```python
from build123d import *

# Parameters (mm, degrees)
SKETCH1_R           = 15
BOSS_EXTRUDE1_DEPTH = 15
SKETCH2_W           = 2.7
SKETCH2_H           = 7.4
SKETCH2_W_2         = 1.7
SKETCH2_H_2         = 6.4
CUT_EXTRUDE1_DEPTH  = 5


with BuildPart() as part:
    # Sketch1 → Boss-Extrude1 (new body)
    with BuildSketch(Plane(origin=(0, 0, 0), x_dir=(1, 0, 0), z_dir=(0, 1, 0))):
        with Locations(Location((0, 0, 0), (0, 0, 270))):
            Circle(SKETCH1_R)
    extrude(amount=BOSS_EXTRUDE1_DEPTH)

    # Sketch2 → Cut-Extrude1 (cut)
    # profile 1 of 3: a face of its own
    with BuildSketch(Plane.XZ):
        with Locations((-11.35, 0)):
            Rectangle(SKETCH2_W, SKETCH2_H)
        with Locations((-11.35, 0)):
            Rectangle(SKETCH2_W_2, SKETCH2_H_2, mode=Mode.SUBTRACT)
    # profile 2 of 3: a face of its own
    with BuildSketch(Plane.XZ):
        with Locations((-11.35, 0)):
            Rectangle(SKETCH2_W_2, SKETCH2_H_2)
    # profile 3 of 3: a face of its own
    with BuildSketch(Plane.XZ):
        with Locations((11.35, 0)):
            Rectangle(SKETCH2_W, SKETCH2_H)
    extrude(amount=-CUT_EXTRUDE1_DEPTH, mode=Mode.SUBTRACT)


solid = part.part
```
Here's how the part is built. I have some questions about the finished solid (model axes, mm). A direction names the side the tool comes from. Coordinates: 2 decimals unless noted, no trailing zeros. Order: outer loops, then holes, each group sorted by start corner. A loop starts at its lowest first (then second) coordinate and runs counter-clockwise, first axis right, second up. Notation, with made-up numbers: (50.5, -19) - (100.5, -19) arc R34 ccw to (100.5, 16) - close; hole circle Ø1 at (59, 8.25). An arc over 180 degrees is marked (long way). One line per question, with ' | ' between items. Start each with the question number.
1. Which directions (+Z, -Z, +X, -X, +Y, -Y) give clear straight access to the entire face, cutting with the end or side of a thin tool? Please do faces 5 (the flat face through (11, 5, 0)), 6 (the flat face through (0, 15, 0)).
2. If we section it at A-A (y = 3.25): Write out the boundary of the cut face in (x, z).
3. I'm going to push flat-ended pins straight in: pin 1 Ø0.8 at (x, y) = (11.5, 3) entering from +Z; pin 2 Ø2.5 at (y, z) = (2.5, -1) entering from +X; pin 3 Ø0.8 at (x, y) = (11.5, 3) entering from -Z; pin 4 Ø0.8 at (x, z) = (-11.5, 0) entering from -Y. Where does each tip first touch, or does it pass through?
4. If we section it at C-C (y = 5.5): Write out the boundary of the cut face in (x, z), and give its area (3 significant figures).
5. If we mould it in two halves opening along X, with no side actions, what happens to faces 1 (the flat face through (0, 0, 0)), 2 (the flat face through (-12.7, 2, 0)), 3 (the cylindrical face through (0.66, 7.395, -14.985)), 4 (the flat face through (-10, 2, 0))? For each: released by +X, released by -X, zero draft, split by the parting line, or undercut.
6. Please list where these lines run through material, in increasing order: line 1 along X through (y, z) = (3.75, 0.5); line 2 along X through (y, z) = (0.5, -2.75); line 3 along Y through (x, z) = (12.25, -1.75). Write a range as [from, to].
7. If we section it at B-B (z = 0): Write out the boundary of the cut face in (x, y), and give its area (3 significant figures).
8. If we section it at D-D (x = 13.25): Write out the boundary of the cut face in (y, z), and give its area (3 significant figures).
Model answer:
1) face 5: -Y | face 6: +Z, -Z, +X, -X, +Y
2) outline: circle Ø30 at (0, 0); hole (-12.7, -3.7) - (-10, -3.7) - (-10, 3.7) - (-12.7, 3.7) - close; hole (10, -3.7) - (12.7, -3.7) - (12.7, 3.7) - (10, 3.7) - close
3) pin 1: stops at z = 10.09 | pin 2: stops at x = 15 | pin 3: stops at z = -10.09 | pin 4: stops at y = 5
4) outline: circle Ø30 at (0, 0) | area: 707 mm²
5) face 1: zero draft | face 2: undercut | face 3: split by the parting line | face 4: undercut
6) line 1: x = [-14.99, -12.7], [-10, 10], [12.7, 14.99] | line 2: x = [-14.75, -12.7], [-10, 10], [12.7, 14.75] | line 3: y = [5, 15]
7) outline: (-15, 0) - (-12.7, 0) - (-12.7, 5) - (-10, 5) - (-10, 0) - (10, 0) - (10, 5) - (12.7, 5) - (12.7, 0) - (15, 0) - (15, 15) - (-15, 15) - close | area: 423 mm²
8) outline: (0, -7.03) - (15, -7.03) - (15, 7.03) - (0, 7.03) - close | area: 211 mm²
